from build123d import *

# Parameters (mm, degrees)
BOSS_EXTRUDE1_DEPTH = 10.2108
SKETCH2_R           = 2.159
SKETCH2_W           = 6.35
SKETCH2_H           = 6.35
CUT_EXTRUDE1_DEPTH  = 58.542673424
SKETCH3_R           = 4.97205
CUT_EXTRUDE2_DEPTH  = 1.27


with BuildPart() as part:
    # Sketch1 → Boss-Extrude1 (new body)
    with BuildSketch(Plane(origin=(0, 0, 0), x_dir=(1, 0, 0), z_dir=(0, 1, 0))):
        with BuildLine():
            Line((0, 5.55625), (50.8, 5.55625))
            ThreePointArc((50.8, 5.55625), (56.35625, 0), (50.8, -5.55625))
            Line((50.8, -5.55625), (0, -5.55625))
            ThreePointArc((0, -5.55625), (-5.55625, 0), (0, 5.55625))
        make_face()
    extrude(amount=BOSS_EXTRUDE1_DEPTH)

    # Sketch2 → Cut-Extrude1 (cut, through all)
    with BuildSketch(Plane(origin=(0, 10.2108, 0), x_dir=(1, 0, 0), z_dir=(0, 1, 0))):
        with Locations(Location((50.8, 0, 0), (0, 0, 270))):
            Circle(SKETCH2_R)
        Rectangle(SKETCH2_W, SKETCH2_H)
    extrude(amount=-CUT_EXTRUDE1_DEPTH, mode=Mode.SUBTRACT)

    # Sketch3 → Cut-Extrude2 (cut)
    with BuildSketch(Plane(origin=(0, 10.2108, 0), x_dir=(1, 0, 0), z_dir=(0, 1, 0))):
        with Locations(Location((0, 0, 0), (0, 0, 270))):
            Circle(SKETCH3_R)
    cut_extrude2 = extrude(amount=-CUT_EXTRUDE2_DEPTH, mode=Mode.SUBTRACT)

    # Mirror1: Cut-Extrude2 across plane
    add(cut_extrude2.mirror(Plane.ZX.offset(5.1054)), mode=Mode.SUBTRACT)


solid = part.part
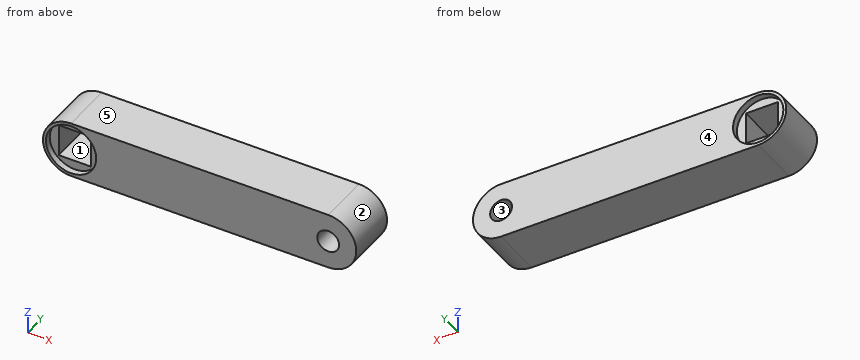
Geometry: final body of the model. Coordinates: model frame, mm. Face numbers are marked on the shaded views. A direction names the side the tool comes from. Give positions to 0.01 mm unless a question says otherwise; leave off trailing zeros. Write each loop counter-clockwise with the first axis right and the second up, starting at its lowest first coordinate (ties: lowest second). Pieces come first, ordered by that corner, then holes.
(1) Mould query, pull axis Z, two halves, no side actions, for the marked faces 3, 4 and 5. Classes: released by +Z, released by -Z, zero draft, split by the parting line, or undercut.
(2) First-contact query: P1, Ø3, axis at x = -2.5, z = -2, coming from the +Y side; P2, Ø6, axis at x = 0, z = 0, coming from the -Y side; P3, Ø4, axis at y = 2.5, z = -3, coming from the +X side. Flat tips, straight axial feed; report the tip coordinate or a pass-through.
(3) Cut plane C-C, the plane z = -3.75. Return loops of the section in (x, y).
(4) Access query for the marked faces 1 and 2. Directions: +Z, -Z, +X, -X, +Y, -Y. A direction counts if a zero-diameter tool reaches every point of the face in a straight line with its end or side. Return the directions, or none.
(5) Ray query, line 1 (X direction, y = 8.25, z = 0) (3 decimals); line 2 (X direction, y = 0.8, z = 0); line 3 (Z direction, x = 51, y = 0.5). Return the intervals inside material, ascending.
(6) Cut plane B-B, the plane z = -0.25. Return loops of the section in (x, y) (3 decimals), then the cut area to 3 significant figures.
(7) Cut plane A-A, the plane y = 2.75. Return loops of the section in (x, z) (1 decimal), then the cut area to 3 significant figures.
Values follow:
1. face 3: undercut
1. face 4: zero draft
1. face 5: released by +Z
2. P1: stops at y = 8.94
2. P2: passes through
2. P3: stops at x = 56.27
3. outline: (-4.1, 0) - (-3.26, 0) - (-3.26, 1.27) - (3.26, 1.27) - (3.26, 0) - (54.9, 0) - (54.9, 10.21) - (3.26, 10.21) - (3.26, 8.94) - (-3.26, 8.94) - (-3.26, 10.21) - (-4.1, 10.21) - close
4. face 1: +Y, -Y
4. face 2: +X, +Y, -Y
5. line 1: x = -5.556 to -3.175, 3.175 to 48.641, 52.959 to 56.356
5. line 2: x = -5.56 to -4.97, 4.97 to 48.64, 52.96 to 56.36
5. line 3: z = -5.55 to -2.15, 2.15 to 5.55
6. outline: (-5.551, 0) - (-4.966, 0) - (-4.966, 1.27) - (-3.175, 1.27) - (-3.175, 8.941) - (-4.966, 8.941) - (-4.966, 10.211) - (-5.551, 10.211) - close; (3.175, 1.27) - (4.966, 1.27) - (4.966, 0) - (48.656, 0) - (48.656, 10.211) - (4.966, 10.211) - (4.966, 8.941) - (3.175, 8.941) - close; (52.944, 0) - (56.351, 0) - (56.351, 10.211) - (52.944, 10.211) - close
6. area: 514 mm2
7. outline: (0, -5.6) - (50.8, -5.6) arc R5.6 ccw to (50.8, 5.6) - (0, 5.6) arc R5.6 ccw to start; hole (-3.2, -3.2) - (3.2, -3.2) - (3.2, 3.2) - (-3.2, 3.2) - close; hole circle Ø4.3 at (50.8, 0)
7. area: 607 mm2
